from build123d import *

# Parameters (mm, degrees)
BOSS_EXTRUDE1_DEPTH = 24


with BuildPart() as part:
    # Sketch2 → Boss-Extrude1 (new body, symmetric)
    with BuildSketch(Plane.XY):
        Polygon((7.5, -2.694744112), (5.366838493, 1), (-5.366838493, 1), (-7.5, -2.694744112), (-6.4, -4.6), (-6, -4.6), (-6, -3.6), (-5, -3.6), (-3.56692895, -1.6), (-3.56692895, -0.6), (-5.2, -0.6), (-5.2, 0), (5.2, 0), (5.2, -0.6), (3.56692895, -0.6), (3.56692895, -1.6), (5, -3.6), (6, -3.6), (6, -4.6), (6.4, -4.6), align=None)
    extrude(amount=BOSS_EXTRUDE1_DEPTH, both=True)


solid = part.part
Read the model definition and answer for the solid it produces. Units are mm, in the model's axes. A direction names the side the tool comes from. Round coordinates to 2 decimals unless told otherwise and drop trailing zeros. Order: outer loops, then holes, each group sorted by start corner. A loop starts at its lowest first (then second) coordinate and runs counter-clockwise, first axis right, second up.
1) The part is cut by section A-A on y = -1.05. Write down the section's boundary in (x, z), plus the area to 3 significant figures.
2) Straight lines are drawn through the part: L1, parallel to X at y = -1.95, z = 9; L2, parallel to X at y = -0.1, z = 4.5; L3, parallel to Y at x = 4.75, z = 8. For each, find the intervals that lie inside material, in ascending order.
3) The mould has two halves that part along Y. Classify faces 4 (the face through (4.273, -2.586, 0.336)), 5 (the face through (-4, -0.6, 0)), 6 (the face through (0, 1, 0)): released by +Y, released by -Y, zero draft, split by the parting line, or undercut.
4) The part is cut by section C-C on x = 1. Write down the section's boundary in (y, z).
5) Flat-ended cylindrical pins translate along their axes: pin 1 (1.5 mm diameter, centred on y = -1.5, z = -3, fed in from +X); pin 2 (0.5 mm diameter, centred on y = -4, z = -3, fed in from -X); pin 3 (1.1 mm diameter, centred on y = -1, z = -7.5, fed in from +X). Find the tip coordinate at first contact, or state that the pin passes through.
6) The part is cut by section B-B on z = -5.5. Write down the section's boundary in (x, y).
7) For faces 1 (the face through (0, 0, 0)), 2 (the face through (-6.418, -0.822, 0.336)), 3 (the face through (3.567, -1, 0)), determine the directions among +Z, -Z, +X, -X, +Y, -Y from which every point of the face is accessible in a straight line to the end or side of a thin tool.
Resolved:
1. outline: (-6.55, -24) - (-3.57, -24) - (-3.57, 24) - (-6.55, 24) - close; (3.57, -24) - (6.55, -24) - (6.55, 24) - (3.57, 24) - close
1. area: 286 mm2
2. L1: x = -7.07 to -3.82, 3.82 to 7.07
2. L2: x = -6 to -5.2, 5.2 to 6
2. L3: y = -3.25 to -0.6, 0 to 1
3. face 4: released by -Y
3. face 5: undercut
3. face 6: released by +Y
4. outline: (0, -24) - (1, -24) - (1, 24) - (0, 24) - close
5. pin 1: stops at x = 7.24
5. pin 2: stops at x = -6.89
5. pin 3: stops at x = 6.84
6. outline: (-7.5, -2.69) - (-6.4, -4.6) - (-6, -4.6) - (-6, -3.6) - (-5, -3.6) - (-3.57, -1.6) - (-3.57, -0.6) - (-5.2, -0.6) - (-5.2, 0) - (5.2, 0) - (5.2, -0.6) - (3.57, -0.6) - (3.57, -1.6) - (5, -3.6) - (6, -3.6) - (6, -4.6) - (6.4, -4.6) - (7.5, -2.69) - (5.37, 1) - (-5.37, 1) - close
7. face 1: +Z, -Z
7. face 2: +Z, -Z, -X, +Y
7. face 3: +Z, -Z, -Y
